Here's how the part is built. I have some questions about the finished solid (model axes, mm). A direction names the side the tool comes from. Round coordinates to 2 decimals unless told otherwise and drop trailing zeros. Write each loop counter-clockwise with the first axis right and the second up, starting at its lowest first coordinate (ties: lowest second). Pieces come first, ordered by that corner, then holes. Notation, with made-up numbers: (71, -31) -> (123, -31) arc R19 cw to (123, 5) -> close; hole circle Ø2 at (62.25, -18.75). An arc over 180 degrees is marked (long way). Answer as CSV lines item,"result".
Autodesk Inventor part; units mm, degrees
ref_plane "YZ Plane" through (0, 0, 0) normal (1, 0, 0) x (0, 1, 0)
ref_plane "XZ Plane" through (0, 0, 0) normal (0, 1, 0) x (-1, 0, 0)
ref_plane "XY Plane" through (0, 0, 0) normal (0, 0, 1) x (1, 0, 0)
sketch "Sketch1" plane through (0, 0, 0) normal (0, 0, 1) x (1, 0, 0)
  line L0 (-22.1155, 0) -> (132.6928, 0)
  line L1 (0, -4.6) -> (0, 6.6)
  line L2 (0, 3) -> (105.6906, 3)
  line L3 (105.6906, 3) -> (105.6906, 5)
  line L4 (105.6906, 5) -> (107.6906, 5)
  line L5 (107.6906, 5) -> (110.5774, 0)
  line L6 (0, 3) -> (3, 0)
  line L7 (0, 3) -> (0, 0)
  line L8 (110, 1) -> (110, 0)
  line L9 (0, -3) -> (3, 0)
  circle A0 centre (78, 0) radius 1.5
  line L10 (2, 3) -> (1, 2)
  line L11 (0, -3) -> (105.6906, -3)
  line L12 (2, -3) -> (1, -2)
  point P0 (1, -2)
  dimension "d0" = 6
  dimension "d2" = 60
  dimension "d3" = 2
  dimension "d4" = 10
  dimension "d5" = 2
  dimension "d6" = 110
  dimension "d10" = 3
  dimension "d14" = 2
  dimension "d16" = 32
revolve "Revolution1" add sketch "Sketch1" angle 360 about axis through (-10, 0, 0) along (1, 0, 0) picked at (78.1773, 0.4675) contours L6 L10 L2 L3 L4 L5 L8 L0 A0 | L2 L10 L6 | A0 L0
extrude "Extrusion1" cut sketch "Sketch1" along normal through all both and the other way through all contours L1 L6 L0 | L0 L9 L1 | L9 L12 L11 | L2 L10 L6 | A0 L0 | L0 A0
properties part number "TW2A-002" material "Steel, Carbon"
Item 1: I need wall thicknesses on L1, parallel to X at y = 0, z = 0.5; L2, parallel to Z at x = 42, y = 0; L3, parallel to X at y = 0, z = 1.75. Which ranges of each line are inside material? Lowest first, please.
Results found:
L1,"x = 3 to 76.5, 79.5 to 110"
L2,"z = -3 to 3"
L3,"x = 3 to 76.5, 79.5 to 109.57"
Item 2: Will these pins go through, and if not, where does the flat tip stop? pin 1 (4 mm diameter, centred on x = 78, y = 0, fed in from -Z); pin 2 (3 mm diameter, centred on x = 93.5, z = -3, fed in from +Y); pin 3 (1 mm diameter, centred on y = 3, z = 0, fed in from -X).
Results found:
pin 1,"stops at z = -3"
pin 2,"stops at y = 2.6"
pin 3,"stops at x = 1.5"
Item 3: For faces 4 (the flat face through (2, -1, 0)), 5 (the cylindrical face through (54.08, 2.86, 0.9)), 6 (the cylindrical face through (106.7, -1.08, -4.88)), which set-ups out of +Z, -Z, +X, -X, +Y, -Y let a thin tool reach every point of the face, with its end or its side?
Results found:
face 4,"+Z, -Z, -X"
face 5,"-X"
face 6,"+X, -X"
Item 4: Suppose I cut it at B-B, the plane x = 16. List the corners of the cut face in (y, z) for me, then the cut area to 3 significant figures.
Results found:
outline,"circle Ø6 at (0, 0)"
area,"28.3 mm²"
Item 5: If we mould it in two halves opening along X, with no side actions, what happens to faces 1 (the conical face through (109.856, -1.249, -0.055)), 2 (the cylindrical face through (78.806, 1.265, 0.042)), 3 (the flat face through (2, 1, 0))? For each: pulls with the +X half, pulls with the -X half, needs draft (parallel to the pull), parting line crosses it, or undercut.
Results found:
face 1,"pulls with the +X half"
face 2,"undercut"
face 3,"pulls with the -X half"
Item 6: Suppose I cut it at C-C, the plane x = 78. List the corners of the cut face in (y, z) for me.
Results found:
outline,"(-1.5, -2.6) -> (-1.5, 2.6) arc R3 ccw to start; (1.5, -2.6) arc R3 ccw to (1.5, 2.6) -> close"
Item 7: Suppose I cut it at A-A, the plane z = 0. List the corners of the cut face in (x, y) for me, then the cut area to 3 significant figures.
Results found:
outline,"(1, -2) -> (2, -3) -> (105.69, -3) -> (105.69, -5) -> (107.69, -5) -> (110, -1) -> (110, 1) -> (107.69, 5) -> (105.69, 5) -> (105.69, 3) -> (2, 3) -> (1, 2) -> (3, 0) -> close; hole circle Ø3 at (78, 0)"
area,"650 mm²"
